from build123d import *

# Parameters (mm, degrees)
SKETCH1_W           = 99
SKETCH1_H           = 79
BOSS_EXTRUDE1_DEPTH = 3
FILLET1_R           = 5
FILLET2_R           = 1
SKETCH2_W           = 110
SKETCH2_H           = 90
BOSS_EXTRUDE2_DEPTH = 2
FILLET3_R           = 5
SKETCH3_W           = 69
SKETCH3_H           = 1
CUT_EXTRUDE1_DEPTH  = 3


with BuildPart() as part:
    # Sketch1 → Boss-Extrude1 (new body)
    with BuildSketch(Plane(origin=(0, 0, 0), x_dir=(1, 0, 0), z_dir=(0, 1, 0))):
        Rectangle(SKETCH1_W, SKETCH1_H)
    extrude(amount=BOSS_EXTRUDE1_DEPTH)

    # Fillet1
    fillet1_edges = [part.edges().sort_by_distance(p)[0] for p in [
        (49.5, 1.5, 39.5),
        (-49.5, 1.5, 39.5),
        (-49.5, 1.5, -39.5),
        (49.5, 1.5, -39.5),
    ]]
    fillet(fillet1_edges, radius=FILLET1_R)

    # Fillet2
    fillet2_edges = [part.edges().sort_by_distance(p)[0] for p in [
        (0, 0, -39.5),
        (49.5, 0, 0),
        (0, 0, 39.5),
        (-49.5, 0, 0),
        (48.035533906, 0, 38.035533906),
        (-48.035533906, 0, 38.035533906),
        (-48.035533906, 0, -38.035533906),
        (48.035533906, 0, -38.035533906),
    ]]
    fillet(fillet2_edges, radius=FILLET2_R)

    # Sketch2 → Boss-Extrude2 (add)
    with BuildSketch(Plane(origin=(0, 3, 0), x_dir=(1, 0, 0), z_dir=(0, 1, 0))):
        Rectangle(SKETCH2_W, SKETCH2_H)
    extrude(amount=BOSS_EXTRUDE2_DEPTH)

    # Fillet3
    fillet3_edges = [part.edges().sort_by_distance(p)[0] for p in [
        (55, 4, 45),
        (55, 4, -45),
        (-55, 4, -45),
        (-55, 4, 45),
    ]]
    fillet(fillet3_edges, radius=FILLET3_R)

    # Sketch3 → Cut-Extrude1 (cut)
    with BuildSketch(Plane(origin=(55, 0, 0), x_dir=(0, 0, -1), z_dir=(1, 0, 0))):
        with Locations((0, 3.5)):
            Rectangle(SKETCH3_W, SKETCH3_H)
    cut_extrude1 = extrude(amount=-CUT_EXTRUDE1_DEPTH, mode=Mode.SUBTRACT)

    # Mirror1: Cut-Extrude1 across plane
    add(cut_extrude1.mirror(Plane(origin=(0, 0, 0), x_dir=(0, 0, 1), z_dir=(1, 0, 0))), mode=Mode.SUBTRACT)


solid = part.part
Read the model definition and answer for the solid it produces. Units are mm, in the model's axes. A direction names the side the tool comes from. Coordinates: 2 decimals unless noted, no trailing zeros. Loops run counter-clockwise (first coordinate to the right, second up) from the corner with the lowest first, then second, coordinate; pieces in that order, holes last. Notation, with made-up numbers: (-28, -24) -> (-15, -24) arc R24 cw to (-15, 11) -> close; hole circle Ø10 at (38, 34). An arc over 180 degrees is marked (long way). Write item = value, one per line. Start each with the question number.
1) The part is cut by section B-B, the plane z = 26.5. Determine the outline of the cut face in (x, y).
2) Given P1, Ø1.6, axis at x = 16, y = 2, coming from the +Z side; P2, Ø0.8, axis at y = 3.5, z = -5, coming from the +X side; P3, Ø1.1, axis at x = -53.5, y = 3.5, coming from the +Z side, each flat-ended and moving along its own axis, determine where each tip first touches the part or whether it passes through.
3) The part is cut by section A-A, the plane x = 13. Determine the outline of the cut face in (y, z).
4) Find the intervals of material crossed by L1, parallel to Z at x = -19, y = 1.8; L2, parallel to X at y = 1.65, z = -29; L3, parallel to Z at x = -47.5, y = 1.25, in increasing order. Write a range as from..to.
5) For faces 1 (the face through (-48.07, 2.01, -38)), 2 (the face through (53, 4, -44)), 3 (the face through (54, 4, 0)), 4 (the face through (48, 2.01, 38.07)), 5 (the face through (-48.07, 2.01, 38)), determine the directions among +Z, -Z, +X, -X, +Y, -Y from which every point of the face is accessible in a straight line to the end or side of a thin tool.
6) The mould has two halves that part along Z. Classify faces 6 (the face through (48.07, 2.01, -38)), 7 (the face through (-1, 5, -1)), 8 (the face through (-54, 4, 0)): pulls with the +Z half, pulls with the -Z half, needs draft (parallel to the pull), parting line crosses it, or undercut.
Result:
q1.outline = (-55, 4) -> (-52, 4) -> (-52, 3) -> (-49.5, 3) -> (-49.5, 1) arc R1 ccw to (-48.5, 0) -> (48.5, 0) arc R1 ccw to (49.5, 1) -> (49.5, 3) -> (52, 3) -> (52, 4) -> (55, 4) -> (55, 5) -> (-55, 5) -> close
q2.P1 = 39.5
q2.P2 = 52
q2.P3 = 44.04
q3.outline = (0, -38.5) arc R1 ccw to (1, -39.5) -> (3, -39.5) -> (3, -45) -> (5, -45) -> (5, 45) -> (3, 45) -> (3, 39.5) -> (1, 39.5) arc R1 ccw to (0, 38.5) -> close
q4.L1 = -39.5..39.5
q4.L2 = -49.5..49.5
q4.L3 = -38.5..38.5
q5.face_1 = -Z, -X, -Y
q5.face_2 = -Z, +X, +Y, -Y
q5.face_3 = +X, -Y
q5.face_4 = +Z, +X, -Y
q5.face_5 = +Z, -X, -Y
q6.face_6 = pulls with the -Z half
q6.face_7 = needs draft
q6.face_8 = undercut
